```python
from build123d import *

# Parameters (mm, degrees)
EXTRUDE_1_DEPTH = 20
FILLET_1_R      = 7
EXTRUDE_2_DEPTH = 20


with BuildPart() as part:
    # 草图1 → 凸台-拉伸1 (new body)
    with BuildSketch(Plane.XY):
        with BuildLine():
            Line((-9.984556, 0.555556), (-19.969112, -178.888889))
            ThreePointArc((-19.969112, -178.888889), (6.717955, -198.837969), (14.75992, -166.503898))
            ThreePointArc((14.75992, -166.503898), (5.273091, -150.735791), (2.641696, -132.522913))
            Line((2.641696, -132.522913), (9.984556, -0.555556))
            ThreePointArc((9.984556, -0.555556), (0.555556, 9.984556), (-9.984556, 0.555556))
        make_face()
    extrude(amount=EXTRUDE_1_DEPTH)

    # 圆角1
    fillet_1_edges = [part.edges().sort_by_distance(p)[0] for p in [
        (6.313126, -66.539235, 20),
        (0.555556, 9.984556, 20),
        (-14.976834, -89.166667, 20),
        (6.717955, -198.837969, 20),
        (-14.976834, -89.166667, 0),
        (0.555556, 9.984556, 0),
        (6.313126, -66.539235, 0),
        (5.273091, -150.735791, 0),
        (6.717955, -198.837969, 0),
        (5.273091, -150.735791, 20),
    ]]
    fillet(fillet_1_edges, radius=FILLET_1_R)

    # 草图2 → 凸台-拉伸2 (add)
    with BuildSketch(Plane.XY):
        with BuildLine():
            Line((5.159577, 28.326291), (9.848078, 1.736482))
            ThreePointArc((9.848078, 1.736482), (1.736482, -9.848078), (-9.848078, -1.736482))
            Line((-9.848078, -1.736482), (-14.536578, 24.853328))
            ThreePointArc((-14.536578, 24.853328), (-6.424983, 36.437887), (5.159577, 28.326291))
        make_face()
    extrude(amount=EXTRUDE_2_DEPTH)


solid = part.part
```
Geometry check sheet. Reference: the model listing, model coordinates, mm. A direction names the side the tool comes from. Give positions to 0.01 mm unless a question says otherwise; leave off trailing zeros. Answer in a Markdown table with one row per item. Add a question column.
Q1. Material ranges on probe 1 along Z at (x, y) = (-6.5, -61); probe 2 along Y at (x, z) = (12.5, 10.5); probe 3 along Y at (x, z) = (14, 4.5), recorded low to high. Write a range as from..to.
Q2. Gauge pin test, flat ends, axial feed: pin 1 (5 mm diameter, centred on x = 2.5, z = 16, fed in from +Y); pin 2 (4 mm diameter, centred on x = 6.5, z = 9, fed in from +Y); pin 3 (12 mm diameter, centred on y = -118.5, z = 4.5, fed in from -X). Record the tip position at first contact, or that the pin passes through.
Q3. Tool access check on faces 1 (the cylindrical face through (-8.94, -4.48, 18.57)), 2 (the cylindrical face through (-8.92, -4.52, 1.38)), 3 (the cylindrical face through (10, 0, 10)). Record the directions out of +Z, -Z, +X, -X, +Y, -Y that give a thin tool (end or side, any length) a straight path to the whole face; none if there is none.
Check values:
| question | item | result |
|---|---|---|
| 1 | probe 1 | z = 0..20 |
| 1 | probe 2 | y = -195.61..-163.84 |
| 1 | probe 3 | y = -193.63..-166.35 |
| 2 | pin 1 | stops at y = 35.42 |
| 2 | pin 2 | stops at y = 30.54 |
| 2 | pin 3 | stops at x = -16.91 |
| 3 | face 1 | +Z, -X |
| 3 | face 2 | -Z, -X |
| 3 | face 3 | +X |
